Autodesk Inventor part; units mm, degrees
ref_plane "YZ Plane" through (0, 0, 0) normal (1, 0, 0) x (0, 1, 0)
ref_plane "XZ Plane" through (0, 0, 0) normal (0, 1, 0) x (-1, 0, 0)
ref_plane "XY Plane" through (0, 0, 0) normal (0, 0, 1) x (1, 0, 0)
sketch "Sketch1" plane through (0, 0, 0) normal (0, 1, 0) x (-1, 0, 0)
  line L0 (-26.4284, 51.2097) -> (59.9316, 51.2097)
  line L1 (31.9916, 28.3497) -> (37.0716, 28.3497)
  line L2 (37.0716, 28.3497) -> (37.0716, 15.6497)
  line L3 (37.0716, 15.6497) -> (31.9916, 15.6497)
  line L4 (31.9916, 15.6497) -> (31.9916, 28.3497)
  line L5 (31.9916, 28.3497) -> (37.0716, 15.6497) construction
  line L6 (37.0716, 28.3497) -> (31.9916, 15.6497) construction
  line L7 (34.5316, 51.2097) -> (34.5316, -7.2103) construction
  line L8 (59.9316, -7.2103) -> (-26.4284, -7.2103) construction
  line L9 (9.1316, 51.2097) -> (9.1316, -7.2103) construction
  line L10 (6.5916, 28.3497) -> (11.6716, 28.3497)
  line L11 (11.6716, 28.3497) -> (11.6716, 15.6497)
  line L12 (11.6716, 15.6497) -> (6.5916, 15.6497)
  line L13 (6.5916, 15.6497) -> (6.5916, 28.3497)
  line L14 (6.5916, 28.3497) -> (11.6716, 15.6497) construction
  line L15 (11.6716, 28.3497) -> (6.5916, 15.6497) construction
  point P0 (0, 0)
  point P1 (34.5316, 21.9997)
  point P2 (34.5316, 21.9997)
  point P3 (9.1316, 21.9997)
  point P4 (9.1316, 21.9997)
  dimension "d4" = 12.7
  dimension "d5" = 5.08
  dimension "d7" = 25.4
extrude "Extrusion1" add sketch "Sketch1" along normal blind 7.62
sketch "Sketch3" plane through (0, 7.62, 0) normal (0, 1, 0) x (1, 0, 0)
  line L0 (-37.0716, -15.6497) -> (-37.0716, -28.3497)
  line L1 (-6.5916, -15.6497) -> (-6.5916, -28.3497)
  line L2 (-37.0716, -15.6497) -> (-6.5916, -15.6497)
  line L3 (-6.5916, -15.6497) -> (-6.5916, -28.3497)
  line L4 (-6.5916, -28.3497) -> (-37.0716, -28.3497)
  line L5 (-37.0716, -28.3497) -> (-37.0716, -15.6497)
  point P0 (0, 0)
extrude "Extrusion2" add sketch "Sketch3" along normal blind 5.08
properties part number "Cpiece"
CAD build for the part. Positions are in the model's coordinates, mm. A direction names the side the tool comes from. Round coordinates to 2 decimals unless told otherwise and drop trailing zeros. Order: outer loops, then holes, each group sorted by start corner. A loop starts at its lowest first (then second) coordinate and runs counter-clockwise, first axis right, second up. Notation, with made-up numbers: (40.25, -16.5) - (67.25, -16.5) arc R25 cw to (67.25, 20.5) - close; hole circle Ø6 at (-2, 59). An arc over 180 degrees is marked (long way). Use CSV: the item, a comma, the result in double quotes. Start each with the question number.
1) Saw through at A-A (y = 5.5). List the corners of the cut face in (x, z).
2) Wall check: L1, parallel to X at y = 7.5, z = 20; L2, parallel to Y at x = -18, z = 22.25. Give the ranges that are in metal, low to high. Write a range as [from, to].
3) Tool access for faces 1 (the flat face through (-31.992, 4, 22)), 2 (the flat face through (-22, 8, 28.35)): list every direction of +Z, -Z, +X, -X, +Y, -Y with a clear straight run to the whole face (end or side of a thin tool).
4) Saw through at B-B (z = 22). List the corners of the cut face in (x, y), and give its area (3 significant figures).
5) Saw through at C-C (x = -20.5). List the corners of the cut face in (y, z).
6) Two-plate mould, pull along X, no slides. Class faces 3 (the flat face through (-37.072, 6, 22)), 4 (the flat face through (-22, 7.62, 22)), 5 (the flat face through (-11.672, 4, 22)), 6 (the flat face through (-34, 0, 22)): pulls with the +X half, pulls with the -X half, needs draft (parallel to the pull), parting line crosses it, or undercut.
Values follow:
1,outline,"(-37.07, 15.65) - (-31.99, 15.65) - (-31.99, 28.35) - (-37.07, 28.35) - close; (-11.67, 15.65) - (-6.59, 15.65) - (-6.59, 28.35) - (-11.67, 28.35) - close"
2,L1,"x = [-37.07, -31.99], [-11.67, -6.59]"
2,L2,"y = [7.62, 12.7]"
3,face 1,"+Z, -Z, -Y"
3,face 2,"+Z, +X, -X, +Y, -Y"
4,outline,"(-37.07, 0) - (-31.99, 0) - (-31.99, 7.62) - (-11.67, 7.62) - (-11.67, 0) - (-6.59, 0) - (-6.59, 12.7) - (-37.07, 12.7) - close"
4,area,"232 mm2"
5,outline,"(7.62, 15.65) - (12.7, 15.65) - (12.7, 28.35) - (7.62, 28.35) - close"
6,face 3,"pulls with the -X half"
6,face 4,"undercut"
6,face 5,"undercut"
6,face 6,"needs draft"
